Input: part model. Units: mm. Frame: model coordinates. A direction names the side the tool comes from. Coordinates: 2 decimals unless noted, no trailing zeros. Loops run counter-clockwise (first coordinate to the right, second up) from the corner with the lowest first, then second, coordinate; pieces in that order, holes last.
(1) Set-up query: faces 4 (the face through (-6.9, 14.4, 0.2)), 5 (the face through (0, 6, -12.5)), 6 (the face through (19, 13.5, -4)). Return all of +Z, -Z, +X, -X, +Y, -Y with unobstructed straight access to the full face (end or side cutting, diameter ignored); none if empty.
(2) Section A-A, the plane x = -19. Return loops of the section in (y, z), then the cut area to 3 significant figures.
(3) Mould query, pull axis X, two halves, no side actions, for faces 1 (the face through (-25, 10, 0)), 2 (the face through (-15.753, 6.844, 0.143)), 3 (the face through (0, 6, 12.5)). Classes: released by +X, released by -X, zero draft, split by the parting line, or undercut.
(4) Section C-C, the plane z = 0. Return loops of the section in (x, y), then the cut area to 4 significant figures.
(5) Section D-D, the plane y = 4.5. Return loops of the section in (x, z).
(6) Contact query for flat-ended pins moving along their axis: P1, Ø4, axis at x = 19, z = 0, coming from the -Y side (3 decimals); P2, Ø0.9, axis at x = 0, z = 5, coming from the +Y side; P3, Ø10, axis at x = -19, z = 0, coming from the +Y side. Output: stop coordinate, or through.
(7) Line query: L1, parallel to X at y = 19, z = 1.75; L2, parallel to X at y = 7.75, z = 1; L3, parallel to Z at x = 19, y = 10. Output: solid intervals per line, ascending.
(8) Section B-B, the plane y = 7.5. Return loops of the section in (x, z), then the cut area to 3 significant figures.
```python
from build123d import *

# Parameters (mm, degrees)
BOSS_EXTRUDE1_DEPTH      = 12.5
BOSS_EXTRUDE1_DEPTH_BACK = 12.5
SKETCH2_R                = 3.25
CUT_EXTRUDE1_DEPTH       = 21
SKETCH3_R                = 5.5
CUT_EXTRUDE2_DEPTH       = 6.5


with BuildPart() as part:
    # Sketch1 → Boss-Extrude1 (new body, two sides)
    with BuildSketch(Plane.XY) as boss_extrude1_sk:
        Polygon((-25, 0), (25, 0), (25, 20), (12.5, 20), (1.5, 9), (1.5, 7), (-1.5, 7), (-1.5, 9), (-12.5, 20), (-25, 20), align=None)
    extrude(amount=BOSS_EXTRUDE1_DEPTH)
    extrude(boss_extrude1_sk.sketch, amount=-BOSS_EXTRUDE1_DEPTH_BACK)

    # Sketch2 → Cut-Extrude1 (cut, through all)
    with BuildSketch(Plane(origin=(0, 20, 0), x_dir=(-1, 0, 0), z_dir=(0, 1, 0))):
        with Locations((19, 0)):
            Circle(SKETCH2_R)
        with Locations((-19, 0)):
            Circle(SKETCH2_R)
    extrude(amount=-CUT_EXTRUDE1_DEPTH, mode=Mode.SUBTRACT)

    # Sketch3 → Cut-Extrude2 (cut)
    with BuildSketch(Plane(origin=(0, 20, 0), x_dir=(-1, 0, 0), z_dir=(0, 1, 0))):
        with Locations((19, 0)):
            Circle(SKETCH3_R)
        with Locations((-19, 0)):
            Circle(SKETCH3_R)
    extrude(amount=-CUT_EXTRUDE2_DEPTH, mode=Mode.SUBTRACT)


solid = part.part
```
Report:
1. face 4: +Z, -Z, +Y
1. face 5: -Z, +X, -X, +Y, -Y
1. face 6: +Y
2. outline: (0, -12.5) - (20, -12.5) - (20, -5.5) - (13.5, -5.5) - (13.5, -3.25) - (0, -3.25) - close; (0, 3.25) - (13.5, 3.25) - (13.5, 5.5) - (20, 5.5) - (20, 12.5) - (0, 12.5) - close
2. area: 341 mm2
3. face 1: released by -X
3. face 2: undercut
3. face 3: zero draft
4. outline: (-25, 0) - (-22.25, 0) - (-22.25, 13.5) - (-24.5, 13.5) - (-24.5, 20) - (-25, 20) - close; (-15.75, 0) - (15.75, 0) - (15.75, 13.5) - (13.5, 13.5) - (13.5, 20) - (12.5, 20) - (1.5, 9) - (1.5, 7) - (-1.5, 7) - (-1.5, 9) - (-12.5, 20) - (-13.5, 20) - (-13.5, 13.5) - (-15.75, 13.5) - close; (22.25, 0) - (25, 0) - (25, 20) - (24.5, 20) - (24.5, 13.5) - (22.25, 13.5) - close
4. area: 521.5 mm2
5. outline: (-25, -12.5) - (25, -12.5) - (25, 12.5) - (-25, 12.5) - close; hole circle Ø6.5 at (-19, 0); hole circle Ø6.5 at (19, 0)
6. P1: passes through
6. P2: stops at y = 7
6. P3: stops at y = 13.5
7. L1: x = -25 to -24.21, -13.79 to -11.5, 11.5 to 13.79, 24.21 to 25
7. L2: x = -25 to -22.09, -15.91 to -1.5, 1.5 to 15.91, 22.09 to 25
7. L3: z = -12.5 to -3.25, 3.25 to 12.5
8. outline: (-25, -12.5) - (-1.5, -12.5) - (-1.5, 12.5) - (-25, 12.5) - close; (1.5, -12.5) - (25, -12.5) - (25, 12.5) - (1.5, 12.5) - close; hole circle Ø6.5 at (-19, 0); hole circle Ø6.5 at (19, 0)
8. area: 1,110 mm2
